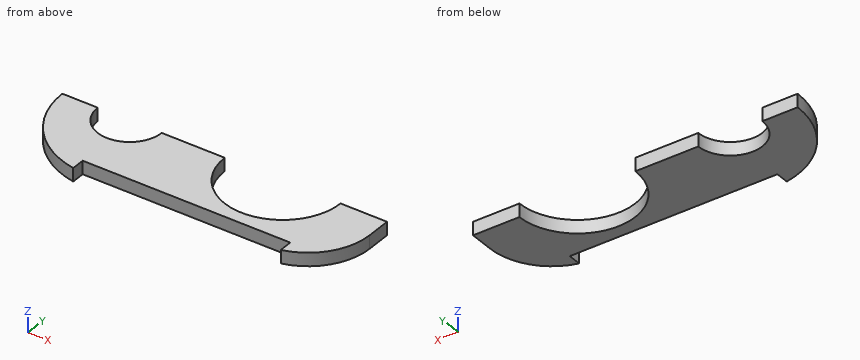
Autodesk Inventor part; units mm, degrees
ref_plane "YZ Plane" through (0, 0, 0) normal (1, 0, 0) x (0, 1, 0)
ref_plane "XZ Plane" through (0, 0, 0) normal (0, 1, 0) x (-1, 0, 0)
ref_plane "XY Plane" through (0, 0, 0) normal (0, 0, 1) x (1, 0, 0)
sketch "Sketch1" plane through (0, 0, 0) normal (0, 0, 1) x (1, 0, 0)
  line L0 (0, 101.6) -> (50.8, 101.6)
  line L1 (466.725, 101.6) -> (466.725, 66.675)
  line L2 (466.725, 0) -> (400.05, 0) construction
  line L3 (0, 0) -> (0, 101.6) construction
  arc A0 (50.8, 101.6) -> (142.875, 101.6) centre (96.8375, 101.6) ccw
  arc A1 (233.3625, 101.6) -> (400.05, 101.6) centre (316.7062, 101.6) ccw
  line L4 (50.8, 101.6) -> (142.875, 101.6) construction
  line L5 (142.875, 101.6) -> (233.3625, 101.6)
  line L6 (233.3625, 101.6) -> (400.05, 101.6) construction
  line L7 (400.05, 101.6) -> (466.725, 101.6)
  arc A2 (0, 101.6) -> (101.6, 0) centre (101.6, 101.6) ccw
  arc A3 (400.05, 0) -> (466.725, 66.675) centre (400.05, 66.675) ccw
  line L8 (400.05, 0) -> (101.6, 0)
  line L9 (466.725, 66.675) -> (466.725, 0) construction
  line L10 (101.6, 0) -> (0, 0) construction
  dimension "d0" = 466.725
  dimension "d1" = 101.6
  dimension "d2" = 50.8
  dimension "d3" = 90.4875
  dimension "d4" = 66.675
  dimension "d5" = 92.075
  dimension "d6" = 166.6875
extrude "Extrusion1" add sketch "Sketch1" along normal blind 19.05
sketch "Sketch2" plane through (0, 0, 19.05) normal (0, 0, 1) x (1, 0, 0)
  line L0 (101.6, 0) -> (101.6, -19.05)
  arc A0 (0, 101.6) -> (101.6, 0) centre (101.6, 101.6) ccw
  line L1 (400.05, 0) -> (400.05, -19.05)
  arc A1 (400.05, 0) -> (466.725, 66.675) centre (400.05, 66.675) ccw
  arc A2 (400.05, -19.05) -> (466.725, 66.675) centre (378.2786, 66.675) ccw
  line L2 (466.725, 66.675) -> (466.725, 101.6)
  arc A3 (0, 101.6) -> (101.6, -19.05) centre (122.4359, 101.6) ccw
  line L3 (0, 101.6) -> (0, 165.1)
  point P0 (0, 0)
extrude "Extrusion2" add sketch "Sketch2" against normal up to surface (19.05 mm away)
properties part number "cannon support front"
Geometry check sheet. Reference: the model listing, model coordinates, mm. Coordinates: 2 decimals unless noted, no trailing zeros. Order: outer loops, then holes, each group sorted by start corner. A loop starts at its lowest first (then second) coordinate and runs counter-clockwise, first axis right, second up. Notation, with made-up numbers: (19.5, -18) - (51.5, -18) arc R14 ccw to (51.5, -2) - close; hole circle Ø4 at (2.5, -28.5). An arc over 180 degrees is marked (long way). Answer in a Markdown table with one row per item. Add a question column.
1) Cross-section at D-D, the plane x = 60.5. Record the cut outline in (y, z).
2) Cross-section at A-A, the plane y = 86. State how many separate pieces and enclosed holes the cut face has, then the cut area to 3 significant figures.
3) Gauge pin test, flat ends, axial feed: P1, Ø1, axis at y = 37, z = 2, coming from the +X side; P2, Ø9.5, axis at x = 186, z = 12, coming from the -Y side; P3, Ø1, axis at y = 50.5, z = 3, coming from the +X side. Record the tip position at first contact, or that the pin passes through.
4) Material ranges on line 1 along X through (y, z) = (87, 4) (3 decimals); line 2 along Y through (x, z) = (190, 1.5); line 3 along X through (y, z) = (25.5, 17.75), recorded low to high. Write a range as [from, to].
5) Cross-section at B-B, the plane y = -6. Record the cut outline in (x, z), then the cut area to 3 significant figures.
Check result:
| question | item | result |
|---|---|---|
| 1 | outline | (-4.01, 0) - (73.33, 0) - (73.33, 19.05) - (-4.01, 19.05) - close |
| 2 | separate pieces | 3 |
| 2 | enclosed holes | 0 |
| 2 | area | 4,100 mm² |
| 3 | P1 | stops at x = 461.77 |
| 3 | P2 | stops at y = 0 |
| 3 | P3 | stops at x = 465.32 |
| 4 | line 1 | x = [0.874, 53.176], [140.499, 234.651], [398.761, 466.725] |
| 4 | line 2 | y = [0, 101.6] |
| 4 | line 3 | x = [26.52, 282.72], [350.69, 456.56] |
| 5 | outline | (64.02, 0) - (101.6, 0) - (101.6, 19.05) - (64.02, 19.05) - close; (400.05, 0) - (428.69, 0) - (428.69, 19.05) - (400.05, 19.05) - close |
| 5 | area | 1,260 mm² |
